Autodesk Inventor part; units mm, degrees
ref_plane "YZ Plane" through (0, 0, 0) normal (1, 0, 0) x (0, 1, 0)
ref_plane "XZ Plane" through (0, 0, 0) normal (0, 1, 0) x (-1, 0, 0)
ref_plane "XY Plane" through (0, 0, 0) normal (0, 0, 1) x (1, 0, 0)
sketch "Boceto1" plane through (0, 0, 0) normal (1, 0, 0) x (0, 1, 0)
  line L0 (3, 30) -> (0, 30)
  line L1 (0, 30) -> (0, 0)
  line L2 (0, 0) -> (26.3114, -9.5766)
  line L3 (0, 0) -> (28, 0) construction
  line L4 (26.3114, -9.5766) -> (26.3114, -51.5766)
  line L5 (26.3114, -51.5766) -> (6.6152, -55.0495)
  line L6 (6.6152, -55.0495) -> (6.6152, -128.0495)
  line L7 (6.6152, -128.0495) -> (9.6152, -128.0495)
  line L8 (9.6152, -128.0495) -> (9.6152, -57.5668)
  line L9 (6.6152, -55.0495) -> (6.6152, -58.0495)
  line L10 (29.3114, -9.5766) -> (29.3114, -54.0939)
  line L11 (27.3375, -6.7575) -> (3, 2.1006)
  line L12 (3, 2.1006) -> (3, 30)
  line L13 (29.3114, -54.0939) -> (9.6152, -57.5668)
  line L14 (27.3375, -6.7575) -> (29.3114, -7.4759)
  line L15 (29.3114, -9.5766) -> (29.3114, -7.4759)
  dimension "d0" = 3
  dimension "d2" = 28
  dimension "d3" = 20
  dimension "d6" = 100
  dimension "d7" = 73
  dimension "d8" = 3
  dimension "d9" = 3
  dimension "d12" = 3
  dimension "d13" = 3
extrude "Extrusión1" add sketch "Boceto1" along normal blind 40
sketch "Boceto2" plane through (0, 0, 0) normal (0, -1, 0) x (1, 0, 0)
  circle A0 centre (20, 15) radius 2.5
  point P0 (0, 0)
  dimension "d16" = 5
extrude "Extrusión2" cut sketch "Boceto2" against normal blind 3
sketch "Boceto3" plane through (0, 6.6152, -128.0495) normal (0, -1, 0) x (1, 0, 0)
  circle A0 centre (20, 23) radius 2.5
  point P0 (0, 128.0495)
  dimension "d19" = 5
extrude "Extrusión3" cut sketch "Boceto3" against normal blind 3
properties part number "1.2.3.UpperArmLink1"
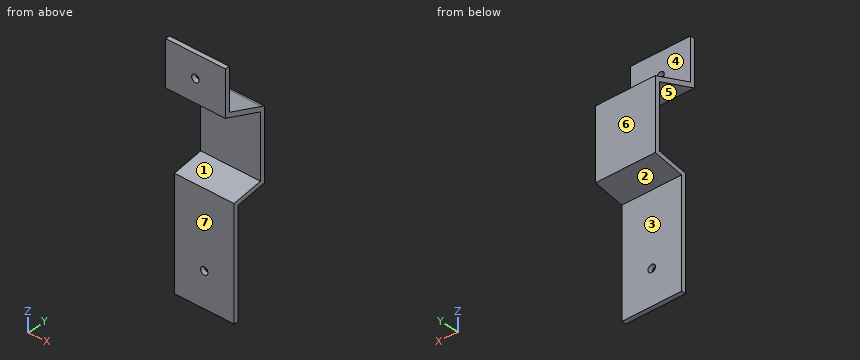
Check sheet for the modelled part. Datum: model origin and axes. Units: mm. Face numbers are marked on the shaded views. A direction names the side the tool comes from. Round coordinates to 2 decimals unless told otherwise and drop trailing zeros. Loops run counter-clockwise (first coordinate to the right, second up) from the corner with the lowest first, then second, coordinate; pieces in that order, holes last. Notation, with made-up numbers: M 15,14.5 L 52,14.5 A23 ccw 52,32.5 Z; hole C 24.5,8 d2. An arc over 180 degrees is marked long. Answer as a JSON object with one key per item and string values.
1. Section check A-A (x = 20). Record the boundary of the cut face in (y, z), plus the area to 3 significant figures.
Reply:
{"outline": "M 0,0 L 26.31,-9.58 L 26.31,-51.58 L 6.62,-55.05 L 6.62,-102.55 L 9.62,-102.55 L 9.62,-57.57 L 29.31,-54.09 L 29.31,-7.48 L 27.34,-6.76 L 3,2.1 L 3,12.5 L 0,12.5 Z; M 0,17.5 L 3,17.5 L 3,30 L 0,30 Z; M 6.62,-128.05 L 9.62,-128.05 L 9.62,-107.55 L 6.62,-107.55 Z", "area": "549 mm²"}
2. Mould release check, pull along Z, two halves, no side actions. Record for the marked faces 1, 2 and 3: pulls with the +Z half, pulls with the -Z half, needs draft (parallel to the pull), parting line crosses it, or undercut.
Reply:
{"face 1": "undercut", "face 2": "pulls with the -Z half", "face 3": "needs draft"}
3. Access from +Z, -Z, +X, -X, +Y, -Y to the whole of each face (thin tool, end or side, straight path). Record for the marked faces 4, 5, 6 and 7.
Reply:
{"face 4": "+Z, +X, -X, +Y", "face 5": "+X, -X, -Y", "face 6": "+Z, -Z, +X, -X, +Y", "face 7": "-Z, +X, -X, -Y"}
4. Scan lines: line 1 (Z direction, x = 20, y = 8.15); line 2 (Z direction, x = 20, y = 7.3); line 3 (Z direction, x = 23, y = 14.5). Record each from-to range of solid material in increasing order.
Reply:
{"line 1": "z = -128.05 to -107.55, -102.55 to -54.78, -2.97 to 0.23", "line 2": "z = -128.05 to -107.55, -102.55 to -54.93, -2.66 to 0.54", "line 3": "z = -56.71 to -53.66, -5.28 to -2.09"}
5. Section check D-D (x = 7.5). Record the boundary of the cut face in (y, z), plus the area to 3 significant figures.
Reply:
{"outline": "M 0,0 L 26.31,-9.58 L 26.31,-51.58 L 6.62,-55.05 L 6.62,-128.05 L 9.62,-128.05 L 9.62,-57.57 L 29.31,-54.09 L 29.31,-7.48 L 27.34,-6.76 L 3,2.1 L 3,30 L 0,30 Z", "area": "579 mm²"}
6. Section check B-B (z = 15). Record the boundary of the cut face in (x, y).
Reply:
{"outline": "M 0,0 L 17.5,0 L 17.5,3 L 0,3 Z; M 22.5,0 L 40,0 L 40,3 L 22.5,3 Z"}
7. Gauge pin test, flat ends, axial feed: P1, Ø6.5, axis at x = 20, z = -105.05, coming from the +Y side; P2, Ø6, axis at x = 20, z = 15, coming from the -Y side; P3, Ø5, axis at x = 34.5, y = 9.5, coming from the +Z side; P4, Ø1.5, axis at x = 11.5, z = -58.5, coming from the -Y side. Record the tip position at first contact, or that the pin passes through.
Reply:
{"P1": "stops at y = 9.62", "P2": "stops at y = 0", "P3": "stops at z = 0.64", "P4": "stops at y = 6.62"}
8. Section check C-C (y = 22.5). Record the boundary of the cut face in (x, z), plus the area to 3 significant figures.
Reply:
{"outline": "M 0,-55.29 L 40,-55.29 L 40,-52.25 L 0,-52.25 Z; M 0,-8.19 L 40,-8.19 L 40,-5 L 0,-5 Z", "area": "250 mm²"}
